CAD build for the part. Positions are in the model's coordinates, mm. A direction names the side the tool comes from. Round coordinates to 2 decimals unless told otherwise and drop trailing zeros. Order: outer loops, then holes, each group sorted by start corner. A loop starts at its lowest first (then second) coordinate and runs counter-clockwise, first axis right, second up. Notation, with made-up numbers: (38, 41.25) - (59, 41.25) arc R28 cw to (59, 60.25) - close; hole circle Ø5 at (55.25, 31). An arc over 180 degrees is marked (long way). Write item = value, one per line.
from build123d import *

# Parameters (mm, degrees)
ESQUISSE1_W         = 32.5
ESQUISSE1_H         = 43
ESQUISSE1_R         = 11.9
BOSS_EXTRU_1_DEPTH  = 12
SKETCH2_W           = 32.5
SKETCH2_H           = 43
BOSS_EXTRUDE1_DEPTH = 5
SKETCH3_R           = 1.5
CUT_EXTRUDE2_DEPTH  = 10
BOSS_EXTRUDE2_DEPTH = 17
SKETCH5_R           = 1.75
CUT_EXTRUDE3_DEPTH  = 48.797930062
SKETCH5_3_R         = 1.75
CUT_EXTRUDE4_DEPTH  = 10


with BuildPart() as part:
    # Esquisse1 → Boss.-Extru.1 (new body)
    with BuildSketch(Plane(origin=(0, 0, 0), x_dir=(1, 0, 0), z_dir=(0, 1, 0))):
        with Locations((0, -14.646640483)):
            Rectangle(ESQUISSE1_W, ESQUISSE1_H)
        with Locations(Location((0, -14.646640483, 0), (0, 0, 270))):
            Circle(ESQUISSE1_R, mode=Mode.SUBTRACT)
    extrude(amount=BOSS_EXTRU_1_DEPTH)

    # Sketch2 → Boss-Extrude1 (add)
    with BuildSketch(Plane(origin=(0, 12, 0), x_dir=(1, 0, 0), z_dir=(0, 1, 0))):
        with Locations((0, -14.646640483)):
            Rectangle(SKETCH2_W, SKETCH2_H)
    extrude(amount=BOSS_EXTRUDE1_DEPTH)

    # Sketch3 → Cut-Extrude2 (cut)
    with BuildSketch(Plane.XY.offset(36.146640483)):
        with Locations((11.25, 10.086854916)):
            Circle(SKETCH3_R)
        with Locations((-6.25, 10.086854916)):
            Circle(SKETCH3_R)
    cut_extrude2 = extrude(amount=-CUT_EXTRUDE2_DEPTH, mode=Mode.SUBTRACT)

    # Mirror1: Cut-Extrude2 across plane
    add(cut_extrude2.mirror(Plane.XY.offset(14.646640483)), mode=Mode.SUBTRACT)

    # Sketch4 → Boss-Extrude2 (add)
    with BuildSketch(Plane(origin=(0, 17, 0), x_dir=(1, 0, 0), z_dir=(0, 1, 0))):
        with BuildLine():
            Line((16.25, -4.646640483), (16.25, -24.646640483))
            ThreePointArc((16.25, -24.646640483), (26.25, -14.646640483), (16.25, -4.646640483))
        make_face()
        with BuildLine():
            Line((-16.25, -4.646640483), (-16.25, -24.646640483))
            ThreePointArc((-16.25, -24.646640483), (-26.25, -14.646640483), (-16.25, -4.646640483))
        make_face()
    extrude(amount=-BOSS_EXTRUDE2_DEPTH)

    # Sketch5 → Cut-Extrude3 (cut, through all)
    with BuildSketch(Plane(origin=(0, 17, 0), x_dir=(1, 0, 0), z_dir=(0, 1, 0))):
        with Locations(Location((-21.25, -14.646640483, 0), (0, 0, 270))):
            Circle(SKETCH5_R)
        with Locations(Location((21.25, -14.646640483, 0), (0, 0, 270))):
            Circle(SKETCH5_R)
    extrude(amount=-CUT_EXTRUDE3_DEPTH, mode=Mode.SUBTRACT)

    # Sketch5<3> → Cut-Extrude4 (cut)
    # profile 1 of 2: a face of its own
    with BuildSketch(Plane(origin=(0, 17, 0), x_dir=(1, 0, 0), z_dir=(0, 1, 0))):
        Polygon((22.924315781, -17.546640483), (24.598631561, -14.646640483), (22.924315781, -11.746640483), (19.575684219, -11.746640483), (17.901368439, -14.646640483), (19.575684219, -17.546640483), align=None)
        with Locations(Location((21.25, -14.646640483, 0), (0, 0, 270))):
            Circle(SKETCH5_3_R, mode=Mode.SUBTRACT)
    # profile 2 of 2: a face of its own
    with BuildSketch(Plane(origin=(0, 17, 0), x_dir=(1, 0, 0), z_dir=(0, 1, 0))):
        Polygon((-19.575684219, -17.546640483), (-22.924315781, -17.546640483), (-24.598631561, -14.646640483), (-22.924315781, -11.746640483), (-19.575684219, -11.746640483), (-17.901368439, -14.646640483), align=None)
        with Locations(Location((-21.25, -14.646640483, 0), (0, 0, 270))):
            Circle(SKETCH5_3_R, mode=Mode.SUBTRACT)
    extrude(amount=-CUT_EXTRUDE4_DEPTH, mode=Mode.SUBTRACT)


solid = part.part
(1) Band-saw the part on A-A on y = 3.75. List the corners of the cut face in (x, z), plus the area to 3 significant figures.
Solved:
outline = (-16.25, -6.85) - (16.25, -6.85) - (16.25, 4.65) arc R10 ccw to (16.25, 24.65) - (16.25, 36.15) - (-16.25, 36.15) - (-16.25, 24.65) arc R10 ccw to (-16.25, 4.65) - close; hole circle Ø3.5 at (-21.25, 14.65); hole circle Ø23.8 at (0, 14.65); hole circle Ø3.5 at (21.25, 14.65)
area = 1,250 mm²
(2) Pull direction Y, two halves, no side cores. Call faces 5 (the cylindrical face through (10.925, 8.623, 31.217)), 6 (the flat face through (0, 12, 14)), 7 (the flat face through (23.75, 12.07, 16.12)): released by +Y, released by -Y, zero draft, split by the parting line, or undercut.
Solved:
face_5 = undercut
face_6 = released by -Y
face_7 = zero draft
(3) Band-saw the part on B-B on x = 0. List the corners of the cut face in (y, z).
Solved:
outline = (0, -6.85) - (17, -6.85) - (17, 36.15) - (0, 36.15) - (0, 26.55) - (12, 26.55) - (12, 2.75) - (0, 2.75) - close
(4) Band-saw the part on C-C on x = 20.5. List the corners of the cut face in (y, z).
Solved:
outline = (0, 5.59) - (17, 5.59) - (17, 11.75) - (7, 11.75) - (7, 13.07) - (0, 13.07) - close; (0, 16.23) - (7, 16.23) - (7, 17.55) - (17, 17.55) - (17, 23.7) - (0, 23.7) - close
(5) Tool access for faces 1 (the flat face through (16.25, 8, -1)), 2 (the flat face through (-16.25, 8, 30)), 3 (the flat face through (23, 7, 16)), 4 (the flat face through (11, 10, 3.147)): list every direction of +Z, -Z, +X, -X, +Y, -Y with a clear straight run to the whole face (end or side of a thin tool).
Solved:
face_1 = -Z, +X, +Y, -Y
face_2 = +Z, -X, +Y, -Y
face_3 = +Y
face_4 = -Z
(6) Drop flat-ended pins along their axis: pin 1 (4.5 mm diameter, centred on x = -21.25, z = 14.65, fed in from +Y); pin 2 (1.8 mm diameter, centred on x = 11.25, y = 10.09, fed in from -Z); pin 3 (2.5 mm diameter, centred on x = -22, y = 11.5, fed in from -Z). Give the stop position or say it passes through.
Solved:
pin_1 = 7
pin_2 = 3.15
pin_3 = 5.72
(7) Band-saw the part on D-D on y = 16. List the corners of the cut face in (x, z), plus the area to 3 significant figures.
Solved:
outline = (-16.25, -6.85) - (16.25, -6.85) - (16.25, 4.65) arc R10 ccw to (16.25, 24.65) - (16.25, 36.15) - (-16.25, 36.15) - (-16.25, 24.65) arc R10 ccw to (-16.25, 4.65) - close; hole (-24.6, 14.65) - (-22.92, 11.75) - (-19.58, 11.75) - (-17.9, 14.65) - (-19.58, 17.55) - (-22.92, 17.55) - close; hole (17.9, 14.65) - (19.58, 11.75) - (22.92, 11.75) - (24.6, 14.65) - (22.92, 17.55) - (19.58, 17.55) - close
area = 1,650 mm²
(8) Probe line 1 along X through (y, z) = (9.25, 2); line 2 along X through (y, z) = (6.75, 15); line 3 along X through (y, z) = (13.5, 14). List the from-to ranges inside material, lowest first.
Solved:
line_1 = -16.25 to -7.49, -5.01 to 10.01, 12.49 to 16.25
line_2 = -26.24 to -22.96, -19.54 to -11.89, 11.89 to 19.54, 22.96 to 26.24
line_3 = -26.23 to -24.23, -18.27 to 18.27, 24.23 to 26.23
